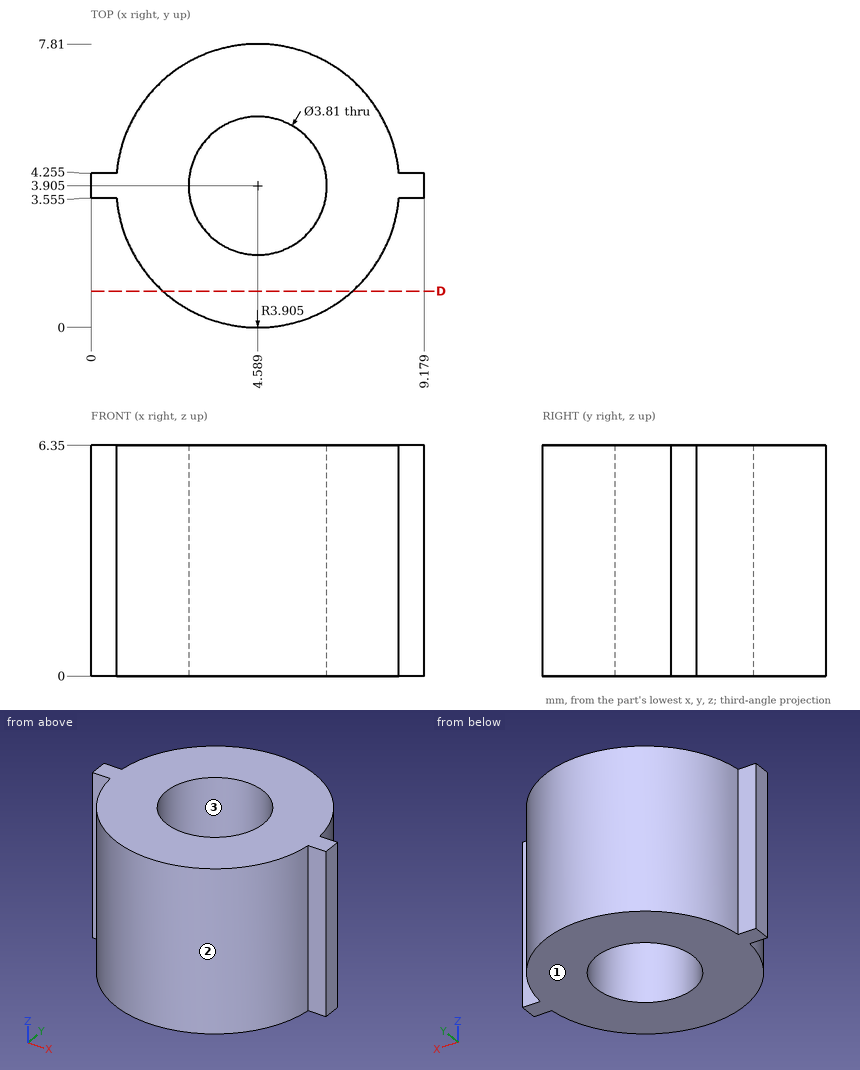
Geometry: see drawing. Coordinates: mm, zero at the bounding-box minimum. Coordinates: 2 decimals unless noted, no trailing zeros. Write each loop counter-clockwise with the first axis right and the second up, starting at its lowest first coordinate (ties: lowest second). Pieces come first, ordered by that corner, then holes.
1) Pin query (flat end, axial travel): pin 1 Ø0.8 at (x, z) = (9, 1.5) entering from +Y (3 decimals); pin 2 Ø2 at (y, z) = (1, 5.5) entering from -X; pin 3 Ø3.5 at (x, y) = (4.59, 3.9) entering from -Z. Return the tip coordinate at first contact, or that it passes through.
2) Material intervals for line 1 along X through (y, z) = (4, 5.75); line 2 along X through (y, z) = (3.25, 3.75); line 3 along Y through (x, z) = (5.5, 5.5), sorted ascending.
3) Section D-D on y = 1. Output: boundary loops of the cut face in (x, z).
4) Mould query, pull axis Y, two halves, no side actions, for the marked faces 1, 2 and 3. Classes: pulls with the +Y half, pulls with the -Y half, needs draft (parallel to the pull), parting line crosses it, or undercut.
Check result:
1. pin 1: stops at y = 4.255
1. pin 2: stops at x = 1.18
1. pin 3: passes through
2. line 1: x = 0 to 2.69, 6.49 to 9.18
2. line 2: x = 0.74 to 2.8, 6.38 to 8.44
2. line 3: y = 0.11 to 2.23, 5.58 to 7.7
3. outline: (1.98, 0) - (7.2, 0) - (7.2, 6.35) - (1.98, 6.35) - close
4. face 1: needs draft
4. face 2: pulls with the -Y half
4. face 3: undercut
